Autodesk Inventor part; units mm, degrees
ref_plane "YZ Plane" through (0, 0, 0) normal (1, 0, 0) x (0, 1, 0)
ref_plane "XZ Plane" through (0, 0, 0) normal (0, 1, 0) x (-1, 0, 0)
ref_plane "XY Plane" through (0, 0, 0) normal (0, 0, 1) x (1, 0, 0)
sketch "Boceto1" plane through (0, 0, 0) normal (1, 0, 0) x (0, 1, 0)
  circle A0 centre (0, 0) radius 2.2
  circle A1 centre (0, 0) radius 3.5
  line L0 (-3.5, 0) -> (16.5, 0)
  circle A2 centre (16.5, 0) radius 2.2
  circle A3 centre (16.5, 0) radius 3.5
  line L1 (2.8723, 2) -> (13.6277, 2)
  line L2 (2.8723, -2) -> (13.6277, -2)
  dimension "d0" = 4.4
  dimension "d1" = 7
  dimension "d2" = 20
  dimension "d3" = 4.4
  dimension "d4" = 7
extrude "Extrusión1" add sketch "Boceto1" along normal blind 5 contours L0 A1 A0 | A0 L0 A1 | L0 A3 L2 A1 | A1 L1 A3 L0 | A3
fillet "Empalme2" radius 1 4 edges at (0, 8.25, -2) (0, 8.25, 2) (0, 20, 0) (0, -3.5, 0)
properties part number "Barra_dedo"
Build history of the part. All positions in model axes, mm. A direction names the side the tool comes from. Round coordinates to 2 decimals unless told otherwise and drop trailing zeros. Write each loop counter-clockwise with the first axis right and the second up, starting at its lowest first coordinate (ties: lowest second). Pieces come first, ordered by that corner, then holes. Notation, with made-up numbers: M 23.25,83 L 54.25,83 A24 cw 54.25,94 Z; hole C 86.25,42.25 d8. An arc over 180 degrees is marked long. Use CSV: the item, a comma, the result in double quotes.
1. Flat gauge pins, fed straight in: pin 1 (3 mm diameter, centred on x = 2.5, y = 10, fed in from -Z); pin 2 (2.5 mm diameter, centred on y = 16.5, z = 0, fed in from -X); pin 3 (2 mm diameter, centred on x = 3, z = 3, fed in from -Y); pin 4 (2 mm diameter, centred on x = 4.5, y = 13.5, fed in from -Z). Where does each tip first touch, or does it go through?
Reply:
pin 1,"stops at z = -2"
pin 2,"passes through"
pin 3,"stops at y = -2.87"
pin 4,"stops at z = -2.87"
2. Saw through at B-B (z = 0). Give the cut face in (x, y), plus the area to 3 significant figures.
Reply:
outline,"M 0,-2.5 A1 ccw 1,-3.5 L 5,-3.5 L 5,-2.2 L 0,-2.2 Z; M 0,2.2 L 5,2.2 L 5,14.3 L 0,14.3 Z; M 0,18.7 L 5,18.7 L 5,20 L 1,20 A1 ccw 0,19 Z"
area,"73.1 mm²"
3. Wall check: probe 1 along Z at (x, y) = (1.7, 0); probe 2 along Y at (x, z) = (3, -1.5); probe 3 along Z at (x, y) = (2.1, 15.5). Give the ranges that are in metal, low to high. Write a range as from..to.
Reply:
probe 1,"z = -3.5..-2.2, 2.2..3.5"
probe 2,"y = -3.16..-1.61, 1.61..14.89, 18.11..19.66"
probe 3,"z = -3.35..-1.96, 1.96..3.35"
4. Tool access for faces 1 (the face through (0.285, 8.333, 1.699)), 2 (the face through (3, 8, -2)), 3 (the face through (0, 8, 0)), 4 (the face through (3, -3.5, -0.1)), 5 (the face through (0.301, 8.333, -1.715)): list every direction of +Z, -Z, +X, -X, +Y, -Y with a clear straight run to the whole face (end or side of a thin tool).
Reply:
face 1,"+Z, -X"
face 2,"-Z, +X, -X"
face 3,"+Z, -Z, -X, +Y, -Y"
face 4,"+X, -X"
face 5,"-Z, -X"
5. Saw through at D-D (y = 5). Give the cut face in (x, z).
Reply:
outline,"M 0,-1 A1 ccw 1,-2 L 5,-2 L 5,2 L 1,2 A1 ccw 0,1 Z"
6. Saw through at A-A (y = 16.5). Give the cut face in (x, z), plus the area to 3 significant figures.
Reply:
outline,"M 0,-2.5 A1 ccw 1,-3.5 L 5,-3.5 L 5,-2.2 L 0,-2.2 Z; M 0,2.2 L 5,2.2 L 5,3.5 L 1,3.5 A1 ccw 0,2.5 Z"
area,"12.6 mm²"
7. Two-plate mould, pull along Y, no slides. Class faces 6 (the face through (2.46, 2.1, -0.66)), 7 (the face through (3, 8, 2)), 8 (the face through (5, 8, 0)): +Y half, -Y half, draft (parallel to the pull), parting line (faces both ways), or undercut.
Reply:
face 6,"undercut"
face 7,"undercut"
face 8,"draft"
8. Saw through at C-C (x = 2.1). Give the cut face in (y, z), plus the area to 3 significant figures.
Reply:
outline,"M 2.87,-2 L 13.63,-2 A3.5 ccw long 13.63,2 L 2.87,2 A3.5 ccw long Z; hole C 0,0 d4.4; hole C 16.5,0 d4.4"
area,"86.2 mm²"
